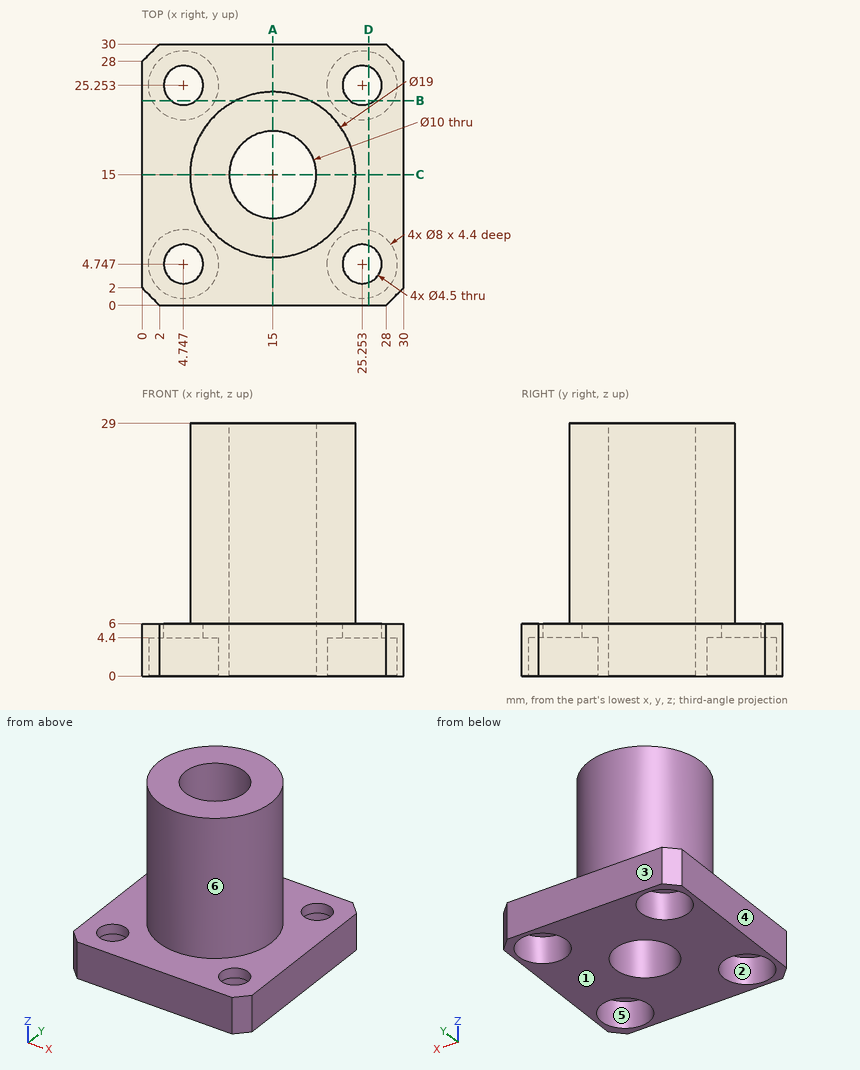
Part print with two shaded views. Sizes in mm from the minimum x, y, z corner. A direction names the side the tool comes from. Coordinates: 2 decimals unless noted, no trailing zeros. Loops run counter-clockwise (first coordinate to the right, second up) from the corner with the lowest first, then second, coordinate; pieces in that order, holes last. Notation, with made-up numbers: (-36.75, 67) -> (-27.75, 67) arc R18 cw to (-27.75, 88) -> close; hole circle Ø2 at (-26.5, -4). An arc over 180 degrees is marked (long way). Answer as a JSON object with one key per item and string values.
Q1. Probe probe 1 along X at (y, z) = (7.75, 2); probe 2 along Y at (x, z) = (7, 2.25); probe 3 along Z at (x, y) = (12.25, 24.25). List the from-to ranges inside material, lowest first.
Report:
{"probe 1": "x = 0 to 2.1, 7.39 to 22.61, 27.9 to 30", "probe 2": "y = 0 to 1.44, 8.05 to 21.95, 28.56 to 30", "probe 3": "z = 0 to 6"}
Q2. Flat gauge pins, fed straight in: P1, Ø8, axis at y = 17, z = 21.5, coming from the +X side; P2, Ø1.5, axis at x = 8, y = 4.5, coming from the +Z side; P3, Ø2.5, axis at x = 23.5, y = 5.5, coming from the -Z side. Where does each tip first touch, or does it go through?
Report:
{"P1": "stops at x = 24.5", "P2": "stops at z = 6", "P3": "stops at z = 4.4"}
Q3. Cut at A-A (x = 15). List the corners of the cut face in (y, z), and give its area (3 significant figures).
Report:
{"outline": "(0, 0) -> (10, 0) -> (10, 29) -> (5.5, 29) -> (5.5, 6) -> (0, 6) -> close; (20, 0) -> (30, 0) -> (30, 6) -> (24.5, 6) -> (24.5, 29) -> (20, 29) -> close", "area": "327 mm2"}
Q4. Cut at B-B (y = 23.5). List the corners of the cut face in (x, z), and give its area (3 significant figures).
Report:
{"outline": "(0, 0) -> (1.15, 0) -> (1.15, 4.4) -> (3.34, 4.4) -> (3.34, 6) -> (0, 6) -> close; (6.16, 4.4) -> (8.34, 4.4) -> (8.34, 0) -> (21.66, 0) -> (21.66, 4.4) -> (23.84, 4.4) -> (23.84, 6) -> (19.24, 6) -> (19.24, 29) -> (10.76, 29) -> (10.76, 6) -> (6.16, 6) -> close; (26.66, 4.4) -> (28.85, 4.4) -> (28.85, 0) -> (30, 0) -> (30, 6) -> (26.66, 6) -> close", "area": "303 mm2"}
Q5. 3-axis set-ups, long thin cutter, end or side, ignore diameter. For the marked faces 4, 5 and 6: which of +Z, -Z, +X, -X, +Y, -Y reach the whole face in a straight line?
Report:
{"face 4": "+Z, -Z, -X, +Y, -Y", "face 5": "-Z", "face 6": "+Z"}
Q6. Cut at D-D (x = 26). List the corners of the cut face in (y, z).
Report:
{"outline": "(0, 0) -> (0.82, 0) -> (0.82, 4.4) -> (2.62, 4.4) -> (2.62, 6) -> (0, 6) -> close; (6.87, 4.4) -> (8.68, 4.4) -> (8.68, 0) -> (21.32, 0) -> (21.32, 4.4) -> (23.13, 4.4) -> (23.13, 6) -> (6.87, 6) -> close; (27.38, 4.4) -> (29.18, 4.4) -> (29.18, 0) -> (30, 0) -> (30, 6) -> (27.38, 6) -> close"}
Q7. Pull direction Y, two halves, no side cores. Call the marked faces 1, 2 and 3: released by +Y, released by -Y, zero draft, split by the parting line, or undercut.
Report:
{"face 1": "zero draft", "face 2": "undercut", "face 3": "released by +Y"}
